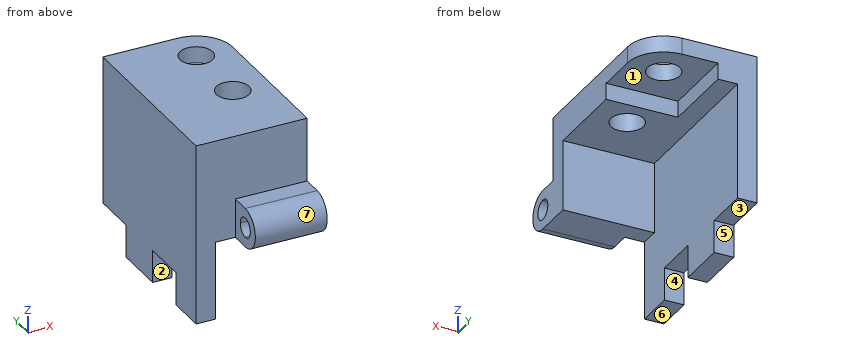
from build123d import *

# Parameters (mm, degrees)
F0_R          = 2.5
F0_W          = 3
F0_H          = 3
F0_W_2        = 14
F1_DEPTH      = 5
F2_DEPTH      = 2.5
F0_H_2        = 21.9
F3_DEPTH      = 22.8
F3_DEPTH_BACK = 5
F4_W          = 3
F4_H          = 7
F5_DEPTH      = 5
F6_DEPTH      = 10.8
F8_DEPTH      = 11


with BuildPart() as f1:
    # F0 (on Top) → F1 (new body)
    with BuildSketch(Plane.XY):
        with BuildLine():
            Line((-5.5, 4.45), (-5.5, 0))
            ThreePointArc((-5.5, 0), (-3.8890872965, -3.8890872965), (0, -5.5))
            ThreePointArc((0, -5.5), (3.8890872965, -3.8890872965), (5.5, 0))
            Line((5.5, 0), (5.5, 4.45))
            Line((5.5, 4.45), (-5.5, 4.45))
        make_face()
        Circle(F0_R, mode=Mode.SUBTRACT)
        with BuildLine():
            Line((-5.5, 5.45), (-5.5, 4.45))
            Line((-5.5, 4.45), (5.5, 4.45))
            Line((5.5, 4.45), (5.5, 10.9))
            ThreePointArc((5.5, 10.9), (3.8890872965, 14.7890872965), (0, 16.4))
            ThreePointArc((0, 16.4), (-3.8890872965, 14.7890872965), (-5.5, 10.9))
            Line((-5.5, 10.9), (-5.5, 5.45))
        make_face()
        with BuildLine():
            ThreePointArc((2.5, 10.9), (0, 8.4), (-2.5, 10.9))
            ThreePointArc((-2.5, 10.9), (0, 13.4), (2.5, 10.9))
        make_face(mode=Mode.SUBTRACT)
        with BuildLine():
            ThreePointArc((0, -5.5), (-3.8890872965, -3.8890872965), (-5.5, 0))
            Line((-5.5, 0), (-5.5, 4.45))
            Line((-5.5, 4.45), (-5.5, 5.45))
            Line((-5.5, 5.45), (-5.5, 10.9))
            Line((-5.5, 10.9), (-5.5, 16.4))
            Line((-5.5, 16.4), (-8.5, 16.4))
            Line((-8.5, 16.4), (-8.5, -5.5))
            Line((-8.5, -5.5), (0, -5.5))
        make_face()
        with BuildLine():
            Line((-5.5, 16.4), (-5.5, 10.9))
            ThreePointArc((-5.5, 10.9), (-3.8890872965, 14.7890872965), (0, 16.4))
            Line((0, 16.4), (-5.5, 16.4))
        make_face()
        with BuildLine():
            ThreePointArc((5.5, 0), (3.8890872965, -3.8890872965), (0, -5.5))
            Line((0, -5.5), (-8.5, -5.5))
            Line((-8.5, -5.5), (-8.5, -8.5))
            Line((-8.5, -8.5), (5.5, -8.5))
            Line((5.5, -8.5), (5.5, 0))
        make_face()
        with Locations((-10, -10)):
            Rectangle(F0_W, F0_H)
        with Locations((-1.5, -10)):
            Rectangle(F0_W_2, F0_H)
    extrude(amount=F1_DEPTH)

    # F0 (on Top) → F2 (cut)
    with BuildSketch(Plane.XY):
        with BuildLine():
            Line((-5.5, 5.45), (-5.5, 4.45))
            Line((-5.5, 4.45), (5.5, 4.45))
            Line((5.5, 4.45), (5.5, 10.9))
            ThreePointArc((5.5, 10.9), (3.8890872965, 14.7890872965), (0, 16.4))
            ThreePointArc((0, 16.4), (-3.8890872965, 14.7890872965), (-5.5, 10.9))
            Line((-5.5, 10.9), (-5.5, 5.45))
        make_face()
        with BuildLine():
            ThreePointArc((2.5, 10.9), (0, 8.4), (-2.5, 10.9))
            ThreePointArc((-2.5, 10.9), (0, 13.4), (2.5, 10.9))
        make_face(mode=Mode.SUBTRACT)
        with BuildLine():
            Line((-5.5, 16.4), (-5.5, 10.9))
            ThreePointArc((-5.5, 10.9), (-3.8890872965, 14.7890872965), (0, 16.4))
            Line((0, 16.4), (-5.5, 16.4))
        make_face()
    extrude(amount=F2_DEPTH, mode=Mode.SUBTRACT)

    # F0 (on Top) → F3 (join, two sides)
    with BuildSketch(Plane.XY) as f3_sk:
        with Locations((-10, -10)):
            Rectangle(F0_W, F0_H)
        with Locations((-10, 5.45)):
            Rectangle(F0_W, F0_H_2)
        with Locations((-10, -7)):
            Rectangle(F0_W, F0_H)
    extrude(amount=-F3_DEPTH)
    extrude(f3_sk.sketch, amount=F3_DEPTH_BACK)

    # F4 (on face) → F5 (cut)
    with BuildSketch(Plane(origin=(0, 0, -22.8), x_dir=(1, 0, 0), z_dir=(0, 0, -1))):
        with Locations((-10, -12.9)):
            Rectangle(F4_W, F4_H)
        with Locations((-10, 2)):
            Rectangle(F4_W, F4_H)
    extrude(amount=-F5_DEPTH, mode=Mode.SUBTRACT)

    # F0 (on Top) → F6 (join)
    with BuildSketch(Plane.XY):
        with Locations((-1.5, -10)):
            Rectangle(F0_W_2, F0_H)
    extrude(amount=-F6_DEPTH)

    # F7 (on face) → F8 (join)
    with BuildSketch(Plane.YZ.offset(5.5)):
        with BuildLine():
            ThreePointArc((-14.5, -4.8), (-17.5, -7.8), (-14.5, -10.8))
            Line((-14.5, -10.8), (-14.5, -9.3))
            ThreePointArc((-14.5, -9.3), (-16, -7.8), (-14.5, -6.3))
            Line((-14.5, -6.3), (-14.5, -4.8))
        make_face()
        with BuildLine():
            Line((-14.5, -9.3), (-14.5, -10.8))
            ThreePointArc((-14.5, -10.8), (-12.3786796564, -9.9213203436), (-11.5, -7.8))
            ThreePointArc((-11.5, -7.8), (-12.3786796564, -5.6786796564), (-14.5, -4.8))
            Line((-14.5, -4.8), (-14.5, -6.3))
            ThreePointArc((-14.5, -6.3), (-13.4393398282, -6.7393398282), (-13, -7.8))
            ThreePointArc((-13, -7.8), (-13.4393398282, -8.8606601718), (-14.5, -9.3))
        make_face()
        with BuildLine():
            ThreePointArc((-14.5, -4.8), (-12.3786796564, -5.6786796564), (-11.5, -7.8))
            Line((-11.5, -7.8), (-11.5, -4.8))
            Line((-11.5, -4.8), (-14.5, -4.8))
        make_face()
        with BuildLine():
            Line((-14.5, -10.8), (-11.5, -10.8))
            Line((-11.5, -10.8), (-11.5, -7.8))
            ThreePointArc((-11.5, -7.8), (-12.3786796564, -9.9213203436), (-14.5, -10.8))
        make_face()
    extrude(amount=-F8_DEPTH)


solid = f1.part
Could you check a few things on this model? Use its own coordinates, in mm. Face numbers are marked on the shaded views. A direction names the side the tool comes from. Coordinates: 2 decimals unless noted, no trailing zeros. Order: outer loops, then holes, each group sorted by start corner. A loop starts at its lowest first (then second) coordinate and runs counter-clockwise, first axis right, second up. Notation, with made-up numbers: (15, 56) -> (55, 56) arc R35 ccw to (55, 91) -> close; hole circle Ø10 at (87.5, -4.5). An arc over 180 degrees is marked (long way). One line per item, written item: value. Start each with the question number.
1) We'd pull the mould along Y, two halves only. Please class the marked faces 4, 5, 6 and 7: +Y half, -Y half, draft (parallel to the pull), parting line (faces both ways), or undercut.
2) Imagine slicing it at C-C on y = -14. List the corners of the cut face in (x, z) for me.
3) I'm going to push flat-ended pins straight in: pin 1 (4 mm diameter, centred on x = 0.5, y = 3, fed in from -Z); pin 2 (0.9 mm diameter, centred on x = -10.5, y = -1.5, fed in from -Z); pin 3 (9 mm diameter, centred on x = 0.5, y = 11, fed in from -Z); pin 4 (6 mm diameter, centred on x = 2, z = -14, fed in from -Y). Where does each tip first touch, or does it pass through?
4) If I drill on L1, parallel to Y at x = 0, z = 3.35; L2, parallel to Y at x = 0, z = 2.05; L3, parallel to Z at x = 4.25, y = -1, over which ranges is the centre line in solid material (lowest first)? Write a range as [from, to].
5) Imagine slicing it at A-A on z = -19.25. List the corners of the cut face in (x, y) for me, plus the area to 3 significant figures.
6) Which directions (+Z, -Z, +X, -X, +Y, -Y) give clear straight access to the entire face, cutting with the end or side of a thin tool? Please do the marked faces 1, 2 and 3.
7) Imagine slicing it at B-B on x = -2. List the corners of the cut face in (y, z) for me.
8) Imagine slicing it at D-D on y = -8. List the corners of the cut face in (x, z) for me.
Answer list:
1. face 4: undercut
1. face 5: +Y half
1. face 6: draft
1. face 7: -Y half
2. outline: (-5.5, -10.8) -> (5.5, -10.8) -> (5.5, -9.21) -> (-5.5, -9.21) -> close; (-5.5, -6.39) -> (5.5, -6.39) -> (5.5, -4.8) -> (-5.5, -4.8) -> close
3. pin 1: stops at z = 0
3. pin 2: stops at z = -17.8
3. pin 3: stops at z = 2.5
3. pin 4: passes through
4. L1: y = [-11.5, -2.5], [2.5, 8.4], [13.4, 16.4]
4. L2: y = [-11.5, -2.5], [2.5, 4.45]
4. L3: z = [0, 5]
5. outline: (-11.5, -11.5) -> (-8.5, -11.5) -> (-8.5, -5.5) -> (-11.5, -5.5) -> close; (-11.5, 1.5) -> (-8.5, 1.5) -> (-8.5, 9.4) -> (-11.5, 9.4) -> close
5. area: 41.7 mm2
6. face 1: -Z, +X, +Y
6. face 2: -Z, +X, -X
6. face 3: -Z, +X, -X, +Y
7. outline: (-14.5, -10.8) -> (-8.5, -10.8) -> (-8.5, 0) -> (-1.5, 0) -> (-1.5, 5) -> (-11.5, 5) -> (-11.5, -4.8) -> (-14.5, -4.8) arc R3 ccw to start; (1.5, 0) -> (4.45, 0) -> (4.45, 2.5) -> (9.4, 2.5) -> (9.4, 5) -> (1.5, 5) -> close; (12.4, 2.5) -> (16.4, 2.5) -> (16.4, 5) -> (12.4, 5) -> close; hole circle Ø3 at (-14.5, -7.8)
8. outline: (-11.5, -22.8) -> (-8.5, -22.8) -> (-8.5, 0) -> (5.5, 0) -> (5.5, 5) -> (-11.5, 5) -> close
